The figure shows three views and two pictorial views of one solid part (mm, origin at its lowest corner). Answer the questions. A direction names the side the tool comes from. Coordinates: 2 decimals unless noted, no trailing zeros. Loops run counter-clockwise (first coordinate to the right, second up) from the corner with the lowest first, then second, coordinate; pieces in that order, holes last. Notation, with made-up numbers: (-10.5, -30.5) - (-6.5, -30.5) arc R12 cw to (-6.5, -19.5) - close; hole circle Ø9 at (-22.5, 42). An arc over 180 degrees is marked (long way). Write each question's results on one line, items separated by ' | '. Start each with the question number.
Item 1: For a pull along X with two mould halves and no side action, classify the marked faces 4, 5 and 6 as +X half, -X half, draft (parallel to the pull), parting line (faces both ways), or undercut.
Item 2: Consider probe 1 along Y at (x, z) = (28, 7.5); probe 2 along Z at (x, y) = (28, 3.5); probe 3 along Y at (x, z) = (16, 2.5). Determine where each line is inside the solid, lowest interval first. Write a range as [from, to].
Item 3: Section B-B, the plane y = 3 is taken. Write down the section's boundary in (x, z), plus the area to 3 significant figures.
Item 4: Section C-C, the plane z = 2.25 is taken. Write down the section's boundary in (x, y), plus the area to 3 significant figures.
Item 5: Section D-D, the plane x = 28 is taken. Write down the section's boundary in (y, z), plus the area to 4 significant figures.
Item 6: Each of these flat-tipped pins is pushed along its axis until it touches: pin 1 Ø10 at (x, y) = (18.5, 10.5) entering from +Z; pin 2 Ø2 at (x, z) = (28.5, 4.5) entering from +Y; pin 3 Ø5 at (x, z) = (28, 7) entering from +Y. Where does it stop, or does it pass through?
Item 7: Section A-A, the plane x = 16 is taken. Write down the section's boundary in (y, z), plus the area to 3 significant figures.
Item 8: A tool of negligible diameter and unlimited length cuts with its end or side. For the marked faces 1, 2 and 3, from which of +Z, -Z, +X, -X, +Y, -Y can it reach the whole face along a straight path? Write none if from no direction.
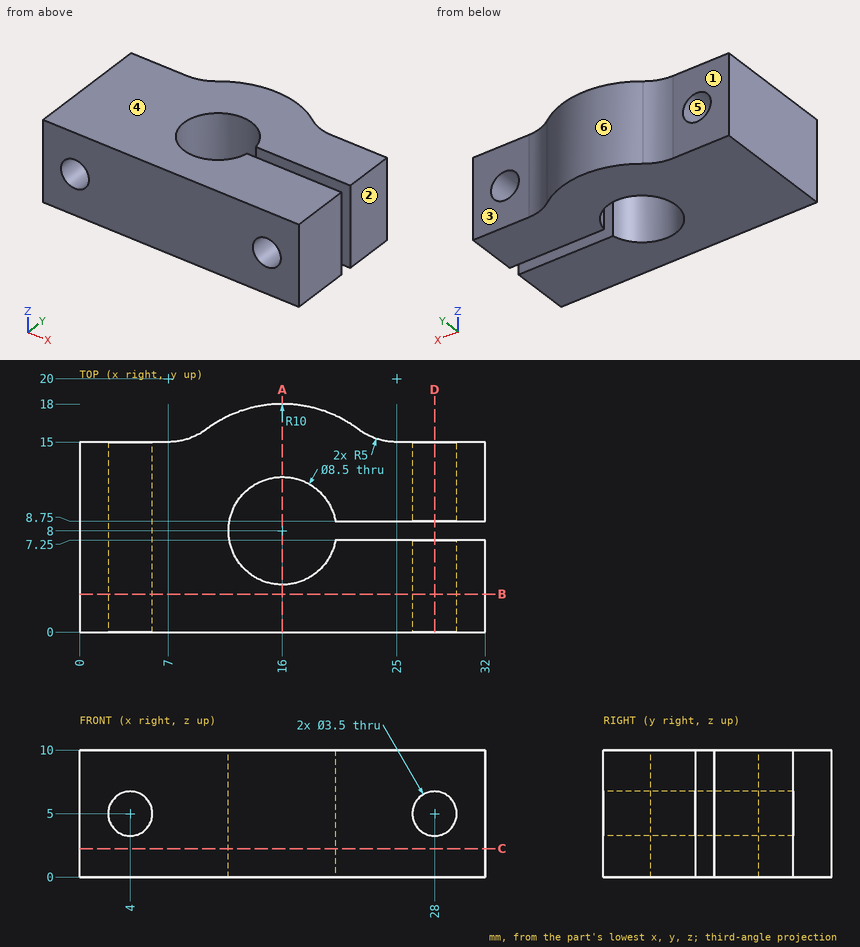
Answer key:
1) face 4: draft | face 5: undercut | face 6: parting line
2) probe 1: y = [0, 7.25], [8.75, 15] | probe 2: z = [0, 3.25], [6.75, 10] | probe 3: y = [0, 3.75], [12.25, 18]
3) outline: (0, 0) - (32, 0) - (32, 10) - (0, 10) - close; hole circle Ø3.5 at (4, 5); hole circle Ø3.5 at (28, 5) | area: 301 mm^2
4) outline: (0, 0) - (32, 0) - (32, 7.25) - (20.18, 7.25) arc R4.25 cw (long way) to (20.18, 8.75) - (32, 8.75) - (32, 15) - (25, 15) arc R5 cw to (22, 16) arc R10 ccw to (10, 16) arc R5 cw to (7, 15) - (0, 15) - close | area: 436 mm^2
5) outline: (0, 0) - (7.25, 0) - (7.25, 3.25) - (0, 3.25) - close; (0, 6.75) - (7.25, 6.75) - (7.25, 10) - (0, 10) - close; (8.75, 0) - (15, 0) - (15, 3.25) - (8.75, 3.25) - close; (8.75, 6.75) - (15, 6.75) - (15, 10) - (8.75, 10) - close | area: 87.75 mm^2
6) pin 1: stops at z = 10 | pin 2: passes through | pin 3: stops at y = 15
7) outline: (0, 0) - (3.75, 0) - (3.75, 10) - (0, 10) - close; (12.25, 0) - (18, 0) - (18, 10) - (12.25, 10) - close | area: 95.0 mm^2
8) face 1: +Z, -Z, -X, +Y | face 2: +Z, -Z, +X, +Y, -Y | face 3: +Z, -Z, +X, +Y
